Here's how the part is built. I have some questions about the finished solid (model axes, mm). Face numbers are marked on the shaded views. A direction names the side the tool comes from. Give positions to 0.01 mm unless a question says otherwise; leave off trailing zeros. Write each loop counter-clockwise with the first axis right and the second up, starting at its lowest first coordinate (ties: lowest second). Pieces come first, ordered by that corner, then holes. Notation, with made-up numbers: (-37.75, 88.25) -> (-11.75, 88.25) arc R31 cw to (-11.75, 127.25) -> close; hole circle Ø2 at (77.5, 67.25). An arc over 180 degrees is marked (long way). Return JSON: item names as keys, results as strings.
from build123d import *

# Parameters (mm, degrees)
EXTRUDE_1_DEPTH      = 27.5
SKETCH_3_W           = 24
SKETCH_3_H           = 24
CUT_EXTRUDE_3_DEPTH  = 24.5
CUT_EXTRUDE_4_DEPTH  = 24.5
SKETCH_7_R           = 3.25
EXTRUDE_4_DEPTH      = 2
SKETCH_10_R          = 3.25
EXTRUDE_5_DEPTH      = 2
CUT_EXTRUDE_6_DEPTH  = 27.5
CUT_EXTRUDE_7_DEPTH  = 3
SKETCH_16_R          = 0.9
CUT_EXTRUDE_10_DEPTH = 6
SKETCH_20_R          = 2.5
EXTRUDE_6_DEPTH      = 5
SKETCH_25_R          = 2.5
EXTRUDE_7_DEPTH      = 5
SKETCH_27_R          = 0.9
CUT_EXTRUDE_13_DEPTH = 6
SKETCH_26_R          = 0.9
CUT_EXTRUDE_14_DEPTH = 6


with BuildPart() as part:
    # 草图1 → 凸台-拉伸1 (new body)
    with BuildSketch(Plane.XY):
        with BuildLine():
            Line((-16.25, -16.25), (16.25, -16.25))
            Line((16.25, -16.25), (16.25, 16.25))
            Line((16.25, 16.25), (-13.25, 16.25))
            ThreePointArc((-13.25, 16.25), (-15.371320344, 15.371320344), (-16.25, 13.25))
            Line((-16.25, 13.25), (-16.25, -16.25))
        make_face()
    extrude(amount=EXTRUDE_1_DEPTH)

    # 草图3 → 切除-拉伸3 (cut)
    with BuildSketch(Plane.XY.offset(27.5)):
        Rectangle(SKETCH_3_W, SKETCH_3_H)
    extrude(amount=-CUT_EXTRUDE_3_DEPTH, mode=Mode.SUBTRACT)

    # 草图4 → 切除-拉伸4 (cut)
    with BuildSketch(Plane.XY.offset(27.5)):
        Polygon((16.25, 16.25), (-7.4, 16.25), (-7.4, 12), (-0.175, 5.8), (16.25, 5.8), align=None)
    cut_extrude_4 = extrude(amount=-CUT_EXTRUDE_4_DEPTH, mode=Mode.SUBTRACT)

    # 镜向1: 切除-拉伸4 across plane
    add(cut_extrude_4.mirror(Plane(origin=(0, 0, 0), x_dir=(0, 0, 1), z_dir=(0.7071067811865477, 0.7071067811865475, 0))), mode=Mode.SUBTRACT)

    # 草图7 → 凸台-拉伸4 (add)
    with BuildSketch(Plane.XZ.offset(16.25)):
        with Locations(Location((6, 9.04, 0), (0, 0, 90))):
            Circle(SKETCH_7_R)
    extrude(amount=EXTRUDE_4_DEPTH)

    # 草图10 → 凸台-拉伸5 (add)
    with BuildSketch(Plane(origin=(16.25, 0, 0), x_dir=(0, 0, -1), z_dir=(1, 0, 0))):
        with Locations(Location((-21.13, -6, 0), (0, 0, 180))):
            Circle(SKETCH_10_R)
    extrude(amount=EXTRUDE_5_DEPTH)

    # 草图13 → 切除-拉伸6 (cut)
    with BuildSketch(Plane.XY.offset(27.5)):
        with BuildLine():
            Line((16.25, -16.25), (9.25, -16.25))
            Line((9.25, -16.25), (9.25, -12))
            ThreePointArc((9.25, -12), (10.055456352, -10.055456352), (12, -9.25))
            Line((12, -9.25), (16.25, -9.25))
            Line((16.25, -9.25), (16.25, -16.25))
        make_face()
    extrude(amount=-CUT_EXTRUDE_6_DEPTH, mode=Mode.SUBTRACT)

    # 草图14 → 切除-拉伸7 (cut)
    with BuildSketch(Plane.XY.offset(3)):
        Polygon((16.25, 5.8), (4.775755008, 5.8), (-7.4, 16.25), (16.25, 16.25), align=None)
    cut_extrude_7 = extrude(amount=-CUT_EXTRUDE_7_DEPTH, mode=Mode.SUBTRACT)

    # 镜向3: 切除-拉伸7 across plane
    add(cut_extrude_7.mirror(Plane(origin=(0, 0, 0), x_dir=(0, 0, 1), z_dir=(0.7071067811865477, 0.7071067811865475, 0))), mode=Mode.SUBTRACT)

    # 草图16 → 切除-拉伸10 (cut)
    with BuildSketch(Plane(origin=(0, 5.8, 0), x_dir=(1, 0, 0), z_dir=(0, 1, 0))):
        with Locations(Location((14.25, -9.04, 0), (0, 0, 180))):
            Circle(SKETCH_16_R)
        with Locations(Location((14.25, -21.03, 0), (0, 0, 180))):
            Circle(SKETCH_16_R)
    cut_extrude_10 = extrude(amount=-CUT_EXTRUDE_10_DEPTH, mode=Mode.SUBTRACT)

    # 镜向4: 切除-拉伸10 across plane
    add(cut_extrude_10.mirror(Plane(origin=(0, 0, 0), x_dir=(0, 0, 1), z_dir=(0.7071067811865477, 0.7071067811865475, 0))), mode=Mode.SUBTRACT)

    # 草图20 → 凸台-拉伸6 (add)
    with BuildSketch(Plane(origin=(18.25, 0, 0), x_dir=(0, 0, -1), z_dir=(1, 0, 0))):
        with Locations((-21.13, -6)):
            Circle(SKETCH_20_R)
    extrude(amount=EXTRUDE_6_DEPTH)

    # 草图25 → 凸台-拉伸7 (add)
    with BuildSketch(Plane.XZ.offset(18.25)):
        with Locations(Location((6, 9.04, 0), (0, 0, 270))):
            Circle(SKETCH_25_R)
    extrude(amount=EXTRUDE_7_DEPTH)

    # 草图27 → 切除-拉伸13 (cut)
    with BuildSketch(Plane(origin=(-7.4, 0, 0), x_dir=(0, 0, -1), z_dir=(1, 0, 0))):
        with Locations((-21.03, 14.25)):
            Circle(SKETCH_27_R)
    extrude(amount=-CUT_EXTRUDE_13_DEPTH, mode=Mode.SUBTRACT)

    # 草图26 → 切除-拉伸14 (cut)
    with BuildSketch(Plane(origin=(0, 7.4, 0), x_dir=(-1, 0, 0), z_dir=(0, -1, 0))):
        with Locations(Location((14.25, -9.04, 0), (0, 0, 180))):
            Circle(SKETCH_26_R)
    extrude(amount=-CUT_EXTRUDE_14_DEPTH, mode=Mode.SUBTRACT)


solid = part.part
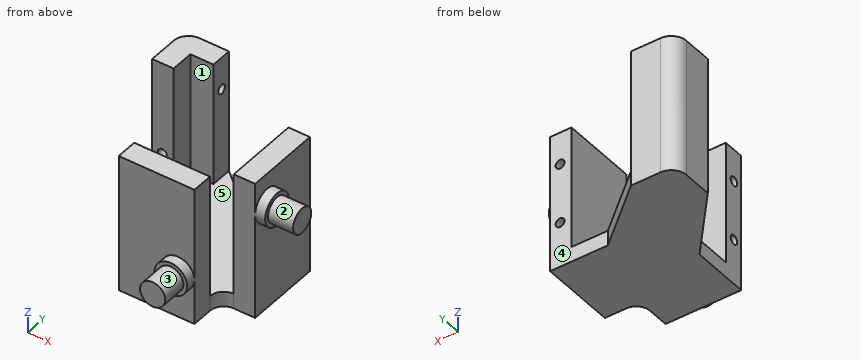
1. Suppose I cut it at D-D, the plane y = 2.5. List the corners of the cut face in (x, z) for me.
Taken from the geometry:
{"outline": "(-12.04, 0) -> (16.25, 0) -> (16.25, 27.5) -> (12, 27.5) -> (12, 3) -> (-12.04, 3) -> close; hole circle Ø1.8 at (14.25, 9.04); hole circle Ø1.8 at (14.25, 21.03)"}
2. Which directions (+Z, -Z, +X, -X, +Y, -Y) give clear straight access to the entire face, cutting with the end or side of a thin tool? Please do the marked faces 1, 2, 3, 4 and 5.
Taken from the geometry:
{"face 1": "+Z, +X, -Y", "face 2": "+X", "face 3": "-Y", "face 4": "+Z, -Z, +X, +Y", "face 5": "+Z"}
3. For pin 1 Ø1.6 at (x, z) = (-14.25, 9.04) entering from -Y; pin 2 Ø3 at (x, z) = (7, 11.5) entering from +Y; pin 3 Ø5.5 at (x, z) = (9.5, 14) entering from +Y; pin 4 Ø10 at (x, y) = (1.5, 4) entering from -Z, each with a flat end and sliding along its axis, tell me the tip position at first contact or that it passes through.
Taken from the geometry:
{"pin 1": "stops at y = 13.4", "pin 2": "stops at y = -12", "pin 3": "stops at y = 5.8", "pin 4": "stops at z = 0"}
4. Suppose I cut it at C-C, the plane x = 14.25. List the corners of the cut face in (y, z) for me, and give its area (3 significant figures).
Taken from the geometry:
{"outline": "(-9.25, 0) -> (5.8, 0) -> (5.8, 8.14) -> (-0.2, 8.14) -> (-0.2, 9.94) -> (5.8, 9.94) -> (5.8, 20.13) -> (-0.2, 20.13) -> (-0.2, 21.93) -> (5.8, 21.93) -> (5.8, 27.5) -> (-9.25, 27.5) -> close", "area": "392 mm²"}
5. Suppose I cut it at B-B, the plane y = -14.25. List the corners of the cut face in (x, z) for me, and give its area (3 significant figures).
Taken from the geometry:
{"outline": "(-5.8, 0) -> (9.25, 0) -> (9.25, 27.5) -> (-5.8, 27.5) -> (-5.8, 21.93) -> (0.2, 21.93) -> (0.2, 20.13) -> (-5.8, 20.13) -> (-5.8, 9.94) -> (0.2, 9.94) -> (0.2, 8.14) -> (-5.8, 8.14) -> close", "area": "392 mm²"}
6. If I drill on line 1 (Y direction, x = -11.35, z = 21.03); line 2 (Z direction, x = -3.5, y = -14.25); line 3 (Z direction, x = -4, y = -14), over which ranges is the centre line in solid material (lowest first)? Write a range as [from, to].
Taken from the geometry:
{"line 1": "y = [12, 13.35], [15.15, 16.25]", "line 2": "z = [0, 8.14], [9.94, 20.13], [21.93, 27.5]", "line 3": "z = [0, 8.18], [9.9, 20.17], [21.89, 27.5]"}
7. Suppose I cut it at A-A, the plane z = 15.5. List the corners of the cut face in (x, y) for me, and give its area (3 significant figures).
Taken from the geometry:
{"outline": "(-16.25, 7.4) -> (-12, 7.4) -> (-12, 12) -> (-7.4, 12) -> (-7.4, 16.25) -> (-13.25, 16.25) arc R3 ccw to (-16.25, 13.25) -> close; (-5.8, -16.25) -> (9.25, -16.25) -> (9.25, -12) -> (-5.8, -12) -> close; (12, -9.25) -> (16.25, -9.25) -> (16.25, 5.8) -> (12, 5.8) -> close", "area": "183 mm²"}
